Part model, mm, in its own coordinate system. A direction names the side the tool comes from. Round coordinates to 2 decimals unless told otherwise and drop trailing zeros. Write each loop counter-clockwise with the first axis right and the second up, starting at its lowest first coordinate (ties: lowest second). Pieces come first, ordered by that corner, then holes. Notation, with made-up numbers: M -36,17.25 L -2,17.25 A29 ccw -2,46.25 Z; hole C 78,-17.5 d8. An arc over 180 degrees is marked long. One line per question, with ' | ' between items. Start each with the question number.
1) Saw through at D-D (x = 0.5). List the corners of the cut face in (y, z), plus the area to 3 significant figures.
2) Saw through at C-C (y = 10.25). List the corners of the cut face in (x, z), plus the area to 3 significant figures.
3) Mould opens along Y. For faces 4 (the face through (-1.58, 1.18, -1.01)), 5 (the face through (0, 7, -0.88)), 6 (the face through (-1.637, 4.482, 0.012)), 7 (the face through (-0.95, 8.96, 0.01)) say: pulls with the +Y half, pulls with the -Y half, needs draft (parallel to the pull), parting line crosses it, or undercut.
4) Drop flat-ended pins along their axis: pin 1 Ø1 at (y, z) = (6.5, 0) entering from +X; pin 2 Ø4 at (x, z) = (-2.5, 4.5) entering from +Y; pin 3 Ø6 at (x, y) = (2, 6.5) entering from -Z; pin 4 Ø2 at (x, z) = (0.5, 1) entering from +Y. Give the stop position or say it passes through.
5) Saw through at B-B (x = -3.5). List the corners of the cut face in (y, z).
6) Saw through at A-A (z = 0). List the corners of the cut face in (x, y) (3 decimals).
7) Wall check: probe 1 along Y at (x, z) = (4.75, 5.5); probe 2 along Y at (x, z) = (0, 1.5); probe 3 along Z at (x, y) = (1, 3.5). Give the ranges that are in metal, low to high. Write a range as [from, to].
8) Tool access for faces 1 (the face through (1.643, 4.518, 0.012)), 2 (the face through (0, 7, 0.88)), 3 (the face through (-2.18, 2.79, 0.29)): list every direction of +Z, -Z, +X, -X, +Y, -Y with a clear straight run to the whole face (end or side of a thin tool).
```python
from build123d import *

# Parameters (mm, degrees)
SKETCH2_W           = 12.5
SKETCH2_H           = 12.5
BOSS_EXTRUDE1_DEPTH = 3
BOSS_EXTRUDE2_DEPTH = 0.88


with BuildPart() as part:
    # Sketch2 → Boss-Extrude1 (new body)
    with BuildSketch(Plane(origin=(0, 0, 0), x_dir=(1, 0, 0), z_dir=(0, 1, 0))):
        Rectangle(SKETCH2_W, SKETCH2_H)
    extrude(amount=-BOSS_EXTRUDE1_DEPTH)

    # Sketch3 → Revolve1 (revolve)
    with BuildSketch(Plane.XY, mode=Mode.PRIVATE) as revolve1_sk:
        Polygon((0, 3.2), (2.2, 3.2), (2.2, 2.4), (1.875, 2.4), (1.875, 0), (0, 0), align=None)
    revolve(revolve1_sk.sketch.rotate(Axis((0, -3, 0), (0, 1, 0)), 90), axis=Axis((0, -3, 0), (0, 1, 0)))

    # Sketch4 → Boss-Extrude2 (add, symmetric)
    with BuildSketch(Plane.XY):
        Polygon((0, 12.2), (1.88, 5.8), (1.4, 3.2), (-1.4, 3.2), (-1.88, 5.8), align=None)
    extrude(amount=BOSS_EXTRUDE2_DEPTH, both=True)


solid = part.part
```
Answer key:
1) outline: M -3,-6.25 L 0,-6.25 L 0,-1.81 L 2.4,-1.81 L 2.4,-2.14 L 3.2,-2.14 L 3.2,-0.88 L 10.5,-0.88 L 10.5,0.88 L 3.2,0.88 L 3.2,2.14 L 2.4,2.14 L 2.4,1.81 L 0,1.81 L 0,6.25 L -3,6.25 Z | area: 62.4 mm2
2) outline: M -0.57,-0.88 L 0.57,-0.88 L 0.57,0.88 L -0.57,0.88 Z | area: 2.02 mm2
3) face 4: undercut | face 5: needs draft | face 6: undercut | face 7: pulls with the +Y half
4) pin 1: stops at x = 1.82 | pin 2: stops at y = 0 | pin 3: stops at z = -0.88 | pin 4: stops at y = 12.2
5) outline: M -3,-6.25 L 0,-6.25 L 0,6.25 L -3,6.25 Z
6) outline: M -6.25,-3 L 6.25,-3 L 6.25,0 L 1.875,0 L 1.875,2.4 L 2.2,2.4 L 2.2,3.2 L 1.4,3.2 L 1.88,5.8 L 0,12.2 L -1.88,5.8 L -1.4,3.2 L -2.2,3.2 L -2.2,2.4 L -1.875,2.4 L -1.875,0 L -6.25,0 Z
7) probe 1: y = [-3, 0] | probe 2: y = [-3, 3.2] | probe 3: z = [-0.88, 0.88]
8) face 1: +Z, -Z, +X | face 2: +Z, +X, -X, +Y | face 3: +Y
